For this review, take the finished solid that the model builds, in its own axes (mm). A direction names the side the tool comes from. Coordinates: 2 decimals unless noted, no trailing zeros. Write each loop counter-clockwise with the first axis right and the second up, starting at its lowest first coordinate (ties: lowest second). Pieces come first, ordered by that corner, then holes. Notation, with made-up numbers: (-25.5, -5) -> (-13.5, -5) arc R5 cw to (-13.5, 4) -> close; hole circle Ø6 at (71, -4.75). An arc over 180 degrees is marked (long way). Put each result on its own line as item: value. Start each with the question number.
Item 1: Insertion check: P1, Ø6.5, axis at x = 11, z = -85.5, coming from the +Y side (3 decimals); P2, Ø8, axis at x = 109, y = 56.5, coming from the +Z side; P3, Ø1.5, axis at x = 71.5, z = -27.5, coming from the +Y side; P4, Ø3.5, axis at x = 6.35, z = -6.35, coming from the -Y side. Each pin has a flat end and moves straight along its axis. Give the tip position at first contact, or say it passes through.
Item 2: To check wall thickness, follow L1, parallel to Z at x = 6, y = 1; L2, parallel to X at y = 1.9, z = -6.35; L3, parallel to X at y = 2.5, z = -82.55. State the ranges of each line that lie inside material, in increasing order.
Item 3: Consider section B-B on x = 58. Give the boundary of the cut face in (y, z), and give its area (3 significant figures).
Item 4: Consider section A-A on y = 20.5. Give the boundary of the cut face in (x, z), and give its area (3 significant figures).
Item 5: For faces 1 (the cylindrical face through (7, 1.6, -4.2)), 2 (the cylindrical face through (116.48, 62.55, -32.2)), 3 (the cylindrical face through (93.41, 54.15, -56.74)), list the 3-axis set-ups (+Z, -Z, +X, -X, +Y, -Y) from which the entire face can be reached by the end or side of a thin tool; tool diameter is ignored.
Item 6: Consider section C-C on z = -68.5. Give the boundary of the cut face in (x, y).
Item 7: The part is to be moulded in two halves that separate along Z. For faces 4 (the flat face through (117.174, 62.756, -44.597)), 5 (the flat face through (49, 15, -88.9)), 6 (the cylindrical face through (116.44, 62.54, -56.74)), 7 (the flat face through (0, 2, -83)), say which applies: +Z half, -Z half, draft (parallel to the pull), parting line (faces both ways), or undercut.
```python
from build123d import *

# Parameters (mm, degrees)
BOSS_EXTRUDE1_DEPTH     = 88.9
SKETCH3_W               = 26.035
SKETCH3_H               = 26.035
CUT_EXTRUDE2_DEPTH      = 74.93
FILLET1_R               = 2.54
CUT_EXTRUDE3_DEPTH      = 164.520153114
CUT_EXTRUDE3_DEPTH_BACK = 164.520153114
FILLET2_R               = 12.7
FILLET3_R               = 12.7
FILLET4_R               = 10.16
CUT_EXTRUDE4_DEPTH      = 164.487937905
CUT_EXTRUDE4_DEPTH_BACK = 164.487937905
SKETCH5_W               = 1.155605494
SKETCH5_H               = 63.5
FILLET5_R               = 5.08
CUT_EXTRUDE5_DEPTH      = 164.487937905
CUT_EXTRUDE5_DEPTH_BACK = 164.487937905
SKETCH6_R               = 2.2479


with BuildPart() as part:
    # Sketch1 → Boss-Extrude1 (new body)
    with BuildSketch(Plane.XY):
        Polygon((0, 0), (38.1, 0), (88.9, 50.8), (122.052919477, 62.866675869), (120.967005522, 65.85019994), (87.152654683, 53.542782743), (36.784871939, 3.175), (0, 3.175), align=None)
    extrude(amount=-BOSS_EXTRUDE1_DEPTH)

    # Sketch3 → Cut-Extrude2 (cut)
    with BuildSketch(Plane(origin=(-5.927480783, 16.285619605, 0), x_dir=(0.9396926207859088, 0.3420201433256679, 0), z_dir=(0.3420201433256679, -0.9396926207859088, 0))):
        with BuildLine():
            Line((103.948597269, -31.59125), (103.948597269, -29.845))
            Line((103.948597269, -29.845), (105.694847269, -29.845))
            ThreePointArc((105.694847269, -29.845), (102.713812052, -28.610214783), (103.948597269, -31.59125))
        make_face()
        with BuildLine():
            Line((105.694847269, -29.845), (103.948597269, -29.845))
            Line((103.948597269, -29.845), (103.948597269, -31.59125))
            ThreePointArc((103.948597269, -31.59125), (105.183382485, -31.079785217), (105.694847269, -29.845))
        make_face()
        with Locations((118.553597269, -44.45)):
            Rectangle(SKETCH3_W, SKETCH3_H)
        with BuildLine():
            ThreePointArc((134.904847269, -29.845), (133.158597269, -28.09875), (131.412347269, -29.845))
            Line((131.412347269, -29.845), (133.158597269, -29.845))
            Line((133.158597269, -29.845), (133.158597269, -31.59125))
            ThreePointArc((133.158597269, -31.59125), (134.393382485, -31.079785217), (134.904847269, -29.845))
        make_face()
        with BuildLine():
            Line((133.158597269, -29.845), (131.412347269, -29.845))
            ThreePointArc((131.412347269, -29.845), (131.923812052, -31.079785217), (133.158597269, -31.59125))
            Line((133.158597269, -31.59125), (133.158597269, -29.845))
        make_face()
        with BuildLine():
            ThreePointArc((134.904847269, -59.055), (134.393382485, -57.820214783), (133.158597269, -57.30875))
            Line((133.158597269, -57.30875), (133.158597269, -59.055))
            Line((133.158597269, -59.055), (131.412347269, -59.055))
            ThreePointArc((131.412347269, -59.055), (133.158597269, -60.80125), (134.904847269, -59.055))
        make_face()
        with BuildLine():
            Line((133.158597269, -59.055), (133.158597269, -57.30875))
            ThreePointArc((133.158597269, -57.30875), (131.923812052, -57.820214783), (131.412347269, -59.055))
            Line((131.412347269, -59.055), (133.158597269, -59.055))
        make_face()
        with BuildLine():
            ThreePointArc((105.694847269, -59.055), (105.183382485, -57.820214783), (103.948597269, -57.30875))
            Line((103.948597269, -57.30875), (103.948597269, -59.055))
            Line((103.948597269, -59.055), (105.694847269, -59.055))
        make_face()
        with BuildLine():
            Line((103.948597269, -59.055), (103.948597269, -57.30875))
            ThreePointArc((103.948597269, -57.30875), (102.713812052, -60.289785217), (105.694847269, -59.055))
            Line((105.694847269, -59.055), (103.948597269, -59.055))
        make_face()
    extrude(amount=-CUT_EXTRUDE2_DEPTH, mode=Mode.SUBTRACT)

    # Fillet1
    fillet1_edges = [part.edges().sort_by_distance(p)[0] for p in [
        (92.70105407, 53.872852754, -31.4325),
        (117.165951452, 62.777347186, -31.4325),
        (117.165951452, 62.777347186, -57.4675),
        (92.70105407, 53.872852754, -57.4675),
    ]]
    fillet(fillet1_edges, radius=FILLET1_R)

    # Sketch4 → Cut-Extrude3 (cut, two sides: drawn at the far end of the back side and taken through both)
    with BuildSketch(Plane(origin=(-5.927480783, 16.285619605, 0), x_dir=(0.9396926207859088, 0.3420201433256679, 0), z_dir=(0.3420201433256679, -0.9396926207859088, 0)).offset(-CUT_EXTRUDE3_DEPTH_BACK)):
        Polygon((136.193897269, -67.6275), (100.913297269, -88.9), (136.193897269, -88.9), align=None)
        Polygon((48.255685329, -12.7), (35.652386673, -12.7), (35.652386673, -76.2), (48.255685329, -76.2), (100.913297269, -44.45), align=None)
        Polygon((121.976342045, -12.7), (136.193897269, -21.2725), (136.193897269, -12.7), align=None)
        Polygon((100.913297269, 0), (121.976342045, -12.7), (136.193897269, -12.7), (136.193897269, 0), align=None)
    extrude(amount=CUT_EXTRUDE3_DEPTH + CUT_EXTRUDE3_DEPTH_BACK, mode=Mode.SUBTRACT)

    # Fillet2
    # the kernel refuses this fillet: 12.7 mm, written as the material it adds along each edge
    with BuildSketch(Plane(origin=(106.909963983, 1.318030631, -44.45), x_dir=(-0.8047299231694688, -0.2928977386570137, -0.5163532370822017), z_dir=(-0.3420201433256679, 0.9396926207859088, 0))) as fillet2_piece_1_section:
        with BuildLine():
            CenterArc((FILLET2_R * 1.65850746269, FILLET2_R), FILLET2_R, 152.175900406, 117.824099594)
            Line((FILLET2_R * 0.774122735992, FILLET2_R * 1.46675866911), (0, 0))
            Line((0, 0), (FILLET2_R * 1.65850746269, 0))
        make_face()
    fillet2_piece_1 = extrude(amount=55.83261194, mode=Mode.PRIVATE)
    fillet2_piece_1 = split(fillet2_piece_1, bisect_by=Plane(origin=(82.567963605, 44.467963605, -44.45), z_dir=(-0.7071067811865475, 0.7071067811865476, 0)), keep=Keep.TOP, mode=Mode.PRIVATE)
    fillet2_piece_1 = split(fillet2_piece_1, bisect_by=Plane(origin=(80.322899575, 46.713027635, -44.45), z_dir=(0.7071067811865475, -0.7071067811865476, 0)), keep=Keep.TOP, mode=Mode.PRIVATE)
    add(fillet2_piece_1)

    # Fillet3
    fillet3_edges = [part.edges().sort_by_distance(p)[0] for p in [
        (36.784871939, 3.175, -6.35),
        (36.784871939, 3.175, -82.55),
    ]]
    fillet(fillet3_edges, radius=FILLET3_R)

    # Fillet4
    fillet4_edges = [part.edges().sort_by_distance(p)[0] for p in [
        (88.357043022, 52.291762035, -88.9),
        (121.509962499, 64.358437904, -67.6275),
        (121.509962499, 64.358437904, -21.2725),
        (88.357043022, 52.291762035, 0),
    ]]
    fillet(fillet4_edges, radius=FILLET4_R)

    # Sketch5 → Cut-Extrude4 (cut, two sides: drawn at the far end of the back side and taken through both)
    with BuildSketch(Plane(origin=(0, 3.175, 0), x_dir=(1, 0, 0), z_dir=(0, 1, 0)).offset(-CUT_EXTRUDE4_DEPTH_BACK)):
        Polygon((36.784871939, 12.7), (36.784871939, 76.2), (31.524359697, 76.2), (0, 76.2), (0, 12.7), (31.524359697, 12.7), align=None)
        with Locations((37.362674686, 44.45)):
            Rectangle(SKETCH5_W, SKETCH5_H)
    extrude(amount=CUT_EXTRUDE4_DEPTH + CUT_EXTRUDE4_DEPTH_BACK, mode=Mode.SUBTRACT)

    # Fillet5
    fillet5_edges = [part.edges().sort_by_distance(p)[0] for p in [
        (0, 1.5875, 0),
        (0, 1.5875, -12.7),
        (0, 1.5875, -76.2),
        (0, 1.5875, -88.9),
    ]]
    fillet(fillet5_edges, radius=FILLET5_R)

    # Sketch6 → Cut-Extrude5 (cut, two sides: drawn at the far end of the back side and taken through both)
    with BuildSketch(Plane(origin=(0, 3.175, 0), x_dir=(1, 0, 0), z_dir=(0, 1, 0)).offset(-CUT_EXTRUDE5_DEPTH_BACK)):
        with Locations(Location((6.35, 82.55, 0), (0, 0, 270))):
            Circle(SKETCH6_R)
        with Locations(Location((25.174359697, 82.55, 0), (0, 0, 270))):
            Circle(SKETCH6_R)
        with Locations(Location((6.35, 6.35, 0), (0, 0, 270))):
            Circle(SKETCH6_R)
        with Locations(Location((25.174359697, 6.35, 0), (0, 0, 270))):
            Circle(SKETCH6_R)
    extrude(amount=CUT_EXTRUDE5_DEPTH + CUT_EXTRUDE5_DEPTH_BACK, mode=Mode.SUBTRACT)


solid = part.part
```
Return value:
1. P1: y = 3.175
1. P2: z = -10.33
1. P3: y = 38.64
1. P4: through
2. L1: -88.9 to -84.77, -80.33 to -76.2, -12.7 to -8.57, -4.13 to 0
2. L2: 0 to 4.1, 8.6 to 22.93, 27.42 to 40
2. L3: 0 to 4.1, 8.6 to 22.93, 27.42 to 40.6
3. outline: (19.9, -88.9) -> (24.39, -88.9) -> (24.39, -67.4) -> (19.9, -68.33) -> close; (19.9, -20.57) -> (24.39, -21.5) -> (24.39, 0) -> (19.9, 0) -> close
3. area: 189 mm^2
4. outline: (54.11, -88.9) -> (58.6, -88.9) -> (58.6, -67.87) -> (54.11, -70.41) -> close; (54.11, -18.49) -> (58.6, -21.03) -> (58.6, 0) -> (54.11, 0) -> close
4. area: 177 mm^2
5. face 1: +Y, -Y
5. face 2: -X, -Y
5. face 3: +X, +Y
6. outline: (56.58, 22.97) -> (57.78, 19.68) -> (88.9, 50.8) -> (119.76, 62.03) -> (118.67, 65.01) -> (87.15, 53.54) -> close
7. face 4: undercut
7. face 5: -Z half
7. face 6: undercut
7. face 7: draft
